from build123d import *

# Parameters (mm, degrees)
BOSS_EXTRUDE1_DEPTH     = 2
SKETCH2_R               = 1.25
CUT_EXTRUDE1_DEPTH      = 2
MIRROR3_COPY_1_SKETCH_R = 1.25
MIRROR3_COPY_1_DEPTH    = 2
FILLET1_R               = 1


with BuildPart() as part:
    # Sketch1 → Boss-Extrude1 (new body)
    with BuildSketch(Plane.XY):
        Polygon((0.767190281, -24.970527522), (9.999292452, -28.813480749), (50.000707548, -28.813480749), (59.232809719, -24.970527522), (60, -15), (60, 0), (0, 0), (0, -15), align=None)
    extrude(amount=BOSS_EXTRUDE1_DEPTH)

    # Sketch2 → Cut-Extrude1 (cut)
    with BuildSketch(Plane(origin=(0, 0, 0), x_dir=(-1, 0, 0), z_dir=(0, 0, -1))):
        with Locations((-4.186666378, -20.978033438)):
            Circle(SKETCH2_R)
    cut_extrude1 = extrude(amount=-CUT_EXTRUDE1_DEPTH, mode=Mode.SUBTRACT)

    # Mirror2: Cut-Extrude1 across plane
    add(cut_extrude1.mirror(Plane(origin=(30, 0, 0), x_dir=(0, 0, 1), z_dir=(1, 0, 0))), mode=Mode.SUBTRACT)

    # Mirror3: Cut-Extrude1 across plane
    add(cut_extrude1.mirror(Plane.ZX.offset(-13.5)), mode=Mode.SUBTRACT)

    # Mirror3 copy 1 sketch → Mirror3 copy 1 (cut)
    with BuildSketch(Plane(origin=(60, -27, 0), x_dir=(1, 0, 0), z_dir=(0, 0, -1))):
        with Locations((-4.186666378, -20.978033438)):
            Circle(MIRROR3_COPY_1_SKETCH_R)
    extrude(amount=-MIRROR3_COPY_1_DEPTH, mode=Mode.SUBTRACT)

    # Fillet1
    fillet1_edges = [part.edges().sort_by_distance(p)[0] for p in [
        (30, 0, 0),
    ]]
    fillet(fillet1_edges, radius=FILLET1_R)


solid = part.part
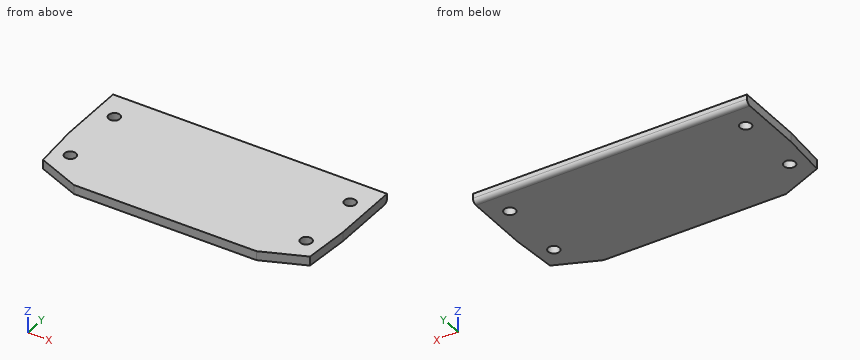
Check sheet for the modelled part. Datum: model origin and axes. Units: mm. Round coordinates to 2 decimals unless told otherwise and drop trailing zeros. Loops run counter-clockwise (first coordinate to the right, second up) from the corner with the lowest first, then second, coordinate; pieces in that order, holes last. Notation, with made-up numbers: M 62.25,13 L 117.25,13 A30 cw 117.25,37 Z; hole C 68.25,-25.75 d3. An arc over 180 degrees is marked long. One line per question, with ' | ' between items. Start each with the question number.
Item 1: Gauge pin test, flat end, axial feed: pin 1 Ø2 at (x, y) = (55.81, -20.98) entering from +Z. Record the tip position at first contact, or that the pin passes through.
Item 2: Section check A-A (x = 55.5). Record the boundary of the cut face in (y, z), and give its area (3 significant figures).
Item 3: Section check C-C (y = -23.75). Record the boundary of the cut face in (x, z), and give its area (3 significant figures).
Item 4: Scan lines: probe 1 along X at (y, z) = (-5.5, 1.35); probe 2 along Y at (x, z) = (3.5, 0.35); probe 3 along X at (y, z) = (-20, 1.5). Record each from-to range of solid material in increasing order.
Item 5: Section check B-B (x = 6.5). Record the boundary of the cut face in (y, z), and give its area (3 significant figures).
Worked out:
1) pin 1: through
2) outline: M -26.52,0 L -22.19,0 L -22.19,2 L -26.52,2 Z; M -19.77,0 L -7.23,0 L -7.23,2 L -19.77,2 Z; M -4.81,0 L -1,0 A1 ccw 0,1 L 0,2 L -4.81,2 Z | area: 43.2 mm^2
3) outline: M 0.67,0 L 59.33,0 L 59.33,2 L 0.67,2 Z | area: 117 mm^2
4) probe 1: 0 to 3.05, 5.32 to 54.68, 56.95 to 60 | probe 2: -26.11 to -22.02, -19.93 to -7.07, -4.98 to -0.24 | probe 3: 0.38 to 3.41, 4.97 to 55.03, 56.59 to 59.62
5) outline: M -27.36,0 L -1,0 A1 ccw 0,1 L 0,2 L -27.36,2 Z | area: 54.5 mm^2
